from build123d import *

# Parameters (mm, degrees)
SKETCH5_W                      = 301.625
SKETCH5_H                      = 1.5875
BASE_FLANGE1_DEPTH             = 381
SKETCH10_W                     = 11.1125
SKETCH10_H                     = 12.7
BOSS_EXTRUDE1_DEPTH            = 1.5875
EDGE_FLANGE1_STRIP_W           = 12.7
EDGE_FLANGE1_STRIP_H           = 1.5875
EDGE_FLANGE1_STRIP_CUT_DEPTH   = 368.3
EDGE_FLANGE1_STRIP_2_W         = 12.7
EDGE_FLANGE1_STRIP_2_H         = 1.5875
EDGE_FLANGE1_STRIP_CUT_2_DEPTH = 368.3
EDGE_FLANGE1_DEPTH             = 368.3
EDGE_FLANGE1_BEND_DEPTH        = 368.3
CUT_EXTRUDE1_START             = -25.4
CUT_EXTRUDE1_DEPTH             = 342.9
EDGE_FLANGE2_STRIP_W           = 11.43
EDGE_FLANGE2_STRIP_H           = 1.5875
EDGE_FLANGE2_STRIP_CUT_DEPTH   = 25.4
EDGE_FLANGE2_DEPTH             = 25.4
EDGE_FLANGE3_STRIP_W           = 11.43
EDGE_FLANGE3_STRIP_H           = 1.5875
EDGE_FLANGE3_STRIP_CUT_DEPTH   = 25.4
EDGE_FLANGE3_DEPTH             = 25.4
FILLET1_R                      = 8
FILLET2_R                      = 3.175
SKETCH30_W                     = 4
SKETCH30_H                     = 1.5875
CUT_EXTRUDE9_DEPTH             = 4
SKETCH31_W                     = 4
SKETCH31_H                     = 1.5875
CUT_EXTRUDE10_DEPTH            = 4
FILLET4_R                      = 1.5


# Sheet-metal steps are written as plain solids
with BuildPart() as part:
    # Sketch5 → Base-Flange1 (new body)
    with BuildSketch(Plane.XY):
        with Locations((0, -0.79375)):
            Rectangle(SKETCH5_W, SKETCH5_H)
    extrude(amount=BASE_FLANGE1_DEPTH)

    # Sketch10 → Boss-Extrude1 (add)
    with BuildSketch(Plane(origin=(0, 0, 0), x_dir=(1, 0, 0), z_dir=(0, 1, 0))):
        with Locations((-156.36875, -6.35)):
            Rectangle(SKETCH10_W, SKETCH10_H)
        with Locations((156.36875, -6.35)):
            Rectangle(SKETCH10_W, SKETCH10_H)
    extrude(amount=-BOSS_EXTRUDE1_DEPTH)

    # Edge-Flange1 strip (across the edge) → Edge-Flange1 strip cut (cut)
    with BuildSketch(Plane(origin=(150.8125, -1.5875, 12.7), x_dir=(-1, 0, 0), z_dir=(0, 0, 1))):
        with Locations((-1.5875, -0.79375)):
            Rectangle(EDGE_FLANGE1_STRIP_W, EDGE_FLANGE1_STRIP_H)
    extrude(amount=EDGE_FLANGE1_STRIP_CUT_DEPTH, mode=Mode.SUBTRACT)

    # Edge-Flange1 strip 2 (across the edge) → Edge-Flange1 strip cut 2 (cut)
    with BuildSketch(Plane(origin=(-150.8125, -1.5875, 381), x_dir=(1, 0, 0), z_dir=(0, 0, -1))):
        with Locations((-1.5875, -0.79375)):
            Rectangle(EDGE_FLANGE1_STRIP_2_W, EDGE_FLANGE1_STRIP_2_H)
    extrude(amount=EDGE_FLANGE1_STRIP_CUT_2_DEPTH, mode=Mode.SUBTRACT)

    # Edge-Flange1 section (across the edge) → Edge-Flange1 (add)
    with BuildSketch(Plane(origin=(150.8125, -1.5875, 12.7), x_dir=(-1, 0, 0), z_dir=(0, 0, 1))):
        with BuildLine():
            Line((0, 3.175), (0, 28.4125))
            Line((0, 28.4125), (1.5875, 28.4125))
            Line((1.5875, 28.4125), (1.5875, 3.175))
            ThreePointArc((1.5875, 3.175), (2.51743597, 0.92993597), (4.7625, 0))
            Line((4.7625, 0), (4.7625, -1.5875))
            ThreePointArc((4.7625, -1.5875), (1.394903955, -0.192596045), (0, 3.175))
        make_face()
    extrude(amount=EDGE_FLANGE1_DEPTH)

    # Edge-Flange1 section 2 (across the edge) → Edge-Flange1 bend (add)
    with BuildSketch(Plane(origin=(-150.8125, -1.5875, 381), x_dir=(1, 0, 0), z_dir=(0, 0, -1))):
        with BuildLine():
            Line((0, 3.175), (0, 28.4125))
            Line((0, 28.4125), (1.5875, 28.4125))
            Line((1.5875, 28.4125), (1.5875, 3.175))
            ThreePointArc((1.5875, 3.175), (2.51743597, 0.92993597), (4.7625, 0))
            Line((4.7625, 0), (4.7625, -1.5875))
            ThreePointArc((4.7625, -1.5875), (1.394903955, -0.192596045), (0, 3.175))
        make_face()
    extrude(amount=EDGE_FLANGE1_BEND_DEPTH)

    # Sketch20 → Cut-Extrude1 (cut)
    with BuildSketch(Plane.XY.offset(381).offset(CUT_EXTRUDE1_START)):
        with BuildLine():
            Line((-150.8125, -4.7625), (-150.8125, -30))
            Line((-150.8125, -30), (-149.225, -30))
            Line((-149.225, -30), (-149.225, -4.7625))
            ThreePointArc((-149.225, -4.7625), (-148.29506403, -2.51743597), (-146.05, -1.5875))
            Line((-146.05, -1.5875), (-146.05, 0))
            ThreePointArc((-146.05, 0), (-149.417596045, -1.394903955), (-150.8125, -4.7625))
        make_face()
        with BuildLine():
            Line((149.225, -4.7625), (149.225, -30))
            Line((149.225, -30), (150.8125, -30))
            Line((150.8125, -30), (150.8125, -4.7625))
            ThreePointArc((150.8125, -4.7625), (149.417596045, -1.394903955), (146.05, 0))
            Line((146.05, 0), (146.05, -1.5875))
            ThreePointArc((146.05, -1.5875), (148.29506403, -2.51743597), (149.225, -4.7625))
        make_face()
    extrude(amount=-CUT_EXTRUDE1_DEPTH, mode=Mode.SUBTRACT)

    # Edge-Flange2 strip (across the edge) → Edge-Flange2 strip cut (cut)
    with BuildSketch(Plane(origin=(-150.8125, -30, 355.6), x_dir=(0, 1, 0), z_dir=(0, 0, 1))):
        with Locations((-1.5875, -0.79375)):
            Rectangle(EDGE_FLANGE2_STRIP_W, EDGE_FLANGE2_STRIP_H)
    extrude(amount=EDGE_FLANGE2_STRIP_CUT_DEPTH, mode=Mode.SUBTRACT)

    # Edge-Flange2 section (across the edge) → Edge-Flange2 (add)
    with BuildSketch(Plane(origin=(-150.8125, -30, 355.6), x_dir=(0, 1, 0), z_dir=(0, 0, 1))):
        with BuildLine():
            Line((0, 2.54), (0, 11.1125))
            Line((0, 11.1125), (1.5875, 11.1125))
            Line((1.5875, 11.1125), (1.5875, 2.54))
            ThreePointArc((1.5875, 2.54), (2.331448776, 0.743948776), (4.1275, 0))
            Line((4.1275, 0), (4.1275, -1.5875))
            ThreePointArc((4.1275, -1.5875), (1.208916761, -0.378583239), (0, 2.54))
        make_face()
    extrude(amount=EDGE_FLANGE2_DEPTH)

    # Edge-Flange3 strip (across the edge) → Edge-Flange3 strip cut (cut)
    with BuildSketch(Plane(origin=(150.8125, -30, 381), x_dir=(0, 1, 0), z_dir=(0, 0, -1))):
        with Locations((-1.5875, -0.79375)):
            Rectangle(EDGE_FLANGE3_STRIP_W, EDGE_FLANGE3_STRIP_H)
    extrude(amount=EDGE_FLANGE3_STRIP_CUT_DEPTH, mode=Mode.SUBTRACT)

    # Edge-Flange3 section (across the edge) → Edge-Flange3 (add)
    with BuildSketch(Plane(origin=(150.8125, -30, 381), x_dir=(0, 1, 0), z_dir=(0, 0, -1))):
        with BuildLine():
            Line((0, 2.54), (0, 11.1125))
            Line((0, 11.1125), (1.5875, 11.1125))
            Line((1.5875, 11.1125), (1.5875, 2.54))
            ThreePointArc((1.5875, 2.54), (2.331448776, 0.743948776), (4.1275, 0))
            Line((4.1275, 0), (4.1275, -1.5875))
            ThreePointArc((4.1275, -1.5875), (1.208916761, -0.378583239), (0, 2.54))
        make_face()
    extrude(amount=EDGE_FLANGE3_DEPTH)

    # Fillet1
    fillet1_edges = [part.edges().sort_by_distance(p)[0] for p in [
        (-146.05, -0.79375, 12.7),
        (146.05, -0.79375, 12.7),
    ]]
    fillet(fillet1_edges, radius=FILLET1_R)

    # Fillet2
    fillet2_edges = [part.edges().sort_by_distance(p)[0] for p in [
        (-161.925, -0.79375, 12.7),
        (-161.925, -0.79375, 0),
        (-161.925, -29.20625, 355.6),
        (-161.925, -29.20625, 381),
        (161.925, -29.20625, 381),
        (161.925, -29.20625, 355.6),
        (161.925, -0.79375, 0),
        (161.925, -0.79375, 12.7),
    ]]
    fillet(fillet2_edges, radius=FILLET2_R)

    # Sketch30 → Cut-Extrude9 (cut)
    with BuildSketch(Plane.ZY.offset(146.05)):
        with Locations((353.6, -0.79375)):
            Rectangle(SKETCH30_W, SKETCH30_H)
    extrude(amount=-CUT_EXTRUDE9_DEPTH, mode=Mode.SUBTRACT)

    # Sketch31 → Cut-Extrude10 (cut)
    with BuildSketch(Plane(origin=(146.05, 0, 0), x_dir=(0, 0, -1), z_dir=(1, 0, 0))):
        with Locations((-353.6, -0.79375)):
            Rectangle(SKETCH31_W, SKETCH31_H)
    extrude(amount=-CUT_EXTRUDE10_DEPTH, mode=Mode.SUBTRACT)

    # Fillet4
    fillet4_edges = [part.edges().sort_by_distance(p)[0] for p in [
        (-146.05, -0.79375, 351.6),
        (-142.05, -0.79375, 351.6),
        (-142.05, -0.79375, 355.6),
        (146.05, -0.79375, 351.6),
        (142.05, -0.79375, 351.6),
        (142.05, -0.79375, 355.6),
    ]]
    fillet(fillet4_edges, radius=FILLET4_R)


solid = part.part
Input: part model. Units: mm. Frame: model coordinates. A direction names the side the tool comes from. Give positions to 0.01 mm unless a question says otherwise; leave off trailing zeros. Order: outer loops, then holes, each group sorted by start corner. A loop starts at its lowest first (then second) coordinate and runs counter-clockwise, first axis right, second up. Notation, with made-up numbers: (12, -22.5) - (38, -22.5) arc R8 ccw to (38, -14.5) - close; hole circle Ø2 at (-32.5, 10.5). An arc over 180 degrees is marked (long way). Write each question's results on one line, items separated by ' | '.
Item 1: Contact query for flat-ended pins moving along their axis: pin 1 Ø4.5 at (x, y) = (149.5, -18) entering from -Z; pin 2 Ø6 at (y, z) = (-5, 80.5) entering from -X; pin 3 Ø0.5 at (x, y) = (156, -1) entering from +Z; pin 4 Ø0.8 at (y, z) = (-1, 210.5) entering from +X. Output: stop coordinate, or through.
A:
pin 1: stops at z = 355.6 | pin 2: passes through | pin 3: stops at z = 12.7 | pin 4: stops at x = 146.05
Item 2: Access query for faces 4 (the flat face through (-158, -28.412, 368)), 5 (the cylindrical face through (-148.456, -0.783, 14.981)), 6 (the cylindrical face through (148.331, -0.805, 15.106)), 7 (the flat face through (149.225, -15, 368)), 8 (the flat face through (158, -28.412, 368)). Directions: +Z, -Z, +X, -X, +Y, -Y. A direction counts if a zero-diameter tool reaches every point of the face in a straight line with its end or side. Return the directions, or none.
A:
face 4: +Z, -Z, -X, +Y | face 5: -X, +Y, -Y | face 6: +X, +Y, -Y | face 7: +Z, -Z, -Y | face 8: +Z, -Z, +X, +Y
Item 3: Draft query along X for faces 1 (the flat face through (-150.6, -16.2, 355.6)), 2 (the flat face through (-150.812, -15, 368)), 3 (the flat face through (-149.225, -15, 368)). Return one class per face: released by +X, released by -X, zero draft, split by the parting line, or undercut.
A:
face 1: zero draft | face 2: released by -X | face 3: undercut
Item 4: Section B-B (x = 103.5). Return loops of the section in (y, z).
A:
outline: (-1.59, 0) - (0, 0) - (0, 381) - (-1.59, 381) - close
Item 5: Section C-C (z = 153). Return loops of the section in (x, y).
A:
outline: (-146.05, -1.59) - (146.05, -1.59) - (146.05, 0) - (-146.05, 0) - close
Item 6: Material intervals for line 1 along Y through (x, z) = (-14.5, 46), sorted ascending.
A:
line 1: y = -1.59 to 0
Item 7: Section A-A (y = -11.5). Return loops of the section in (x, z) (1 decimal).
A:
outline: (-150.8, 355.6) - (-149.2, 355.6) - (-149.2, 381) - (-150.8, 381) - close; (149.2, 355.6) - (150.8, 355.6) - (150.8, 381) - (149.2, 381) - close
